Design review of the part built by this model. Coordinates are the model's own, in mm. A direction names the side the tool comes from. Give positions to 0.01 mm unless a question says otherwise; leave off trailing zeros. Order: outer loops, then holes, each group sorted by start corner. A loop starts at its lowest first (then second) coordinate and runs counter-clockwise, first axis right, second up. Notation, with made-up numbers: (43, 62.25) -> (83, 62.25) arc R23 ccw to (83, 70.25) -> close; hole circle Ø9 at (2, -24). An arc over 180 degrees is marked (long way). Answer in a Markdown table with one row per item. Add a question column.
```python
from build123d import *

# Parameters (mm, degrees)
BOSS_EXTRUDE1_DEPTH  = 60
CUT_EXTRUDE1_DEPTH   = 40
SKETCH11_W           = 2.5
SKETCH11_H           = 2.5
BOSS_EXTRUDE2_DEPTH  = 2.5
SKETCH14_W           = 3
SKETCH14_H           = 60
BOSS_EXTRUDE5_DEPTH  = 47
SKETCH12_R           = 1.125
BOSS_EXTRUDE3_DEPTH  = 6
CUT_EXTRUDE2_DEPTH   = 10
SKETCH16_W           = 100
SKETCH16_H           = 55
BOSS_EXTRUDE6_DEPTH  = 5
BOSS_EXTRUDE8_START  = -2
BOSS_EXTRUDE8_DEPTH  = 16
SKETCH19_W           = 2.25
SKETCH19_H           = 17
BOSS_EXTRUDE9_DEPTH  = 2.5
SKETCH20_W           = 100
SKETCH20_H           = 55
SKETCH20_W_2         = 59
SKETCH20_H_2         = 13.250841504
BOSS_EXTRUDE10_DEPTH = 5


with BuildPart() as part:
    # Sketch1 → Boss-Extrude1 (new body)
    with BuildSketch(Plane(origin=(0, 0, 0), x_dir=(1, 0, 0), z_dir=(0, 1, 0))):
        Polygon((40.01980198, -3.267326733), (40.01980198, 51.732673267), (35.01980198, 51.732673267), (35.01980198, 4.732673267), (-26.98019802, 4.732673267), (-26.98019802, 51.732673267), (-59.98019802, 51.732673267), (-59.98019802, -3.267326733), align=None)
    extrude(amount=BOSS_EXTRUDE1_DEPTH)

    # Sketch3 → Cut-Extrude1 (cut)
    with BuildSketch(Plane.ZY.offset(59.98019802)):
        with BuildLine():
            Line((-28.858094019, 44.125420752), (-51.732673267, 44.125420752))
            Line((-51.732673267, 44.125420752), (-51.732673267, 15.874579248))
            Line((-51.732673267, 15.874579248), (-28.858094019, 15.874579248))
            ThreePointArc((-28.858094019, 15.874579248), (-14.732673267, 30), (-28.858094019, 44.125420752))
        make_face()
    extrude(amount=-CUT_EXTRUDE1_DEPTH, mode=Mode.SUBTRACT)

    # Sketch11 → Boss-Extrude2 (add)
    with BuildSketch(Plane(origin=(0, 0, -14.732673267), x_dir=(-1, 0, 0), z_dir=(0, 0, -1))):
        with Locations((32.98019802, 30)):
            Rectangle(SKETCH11_W, SKETCH11_H)
    extrude(amount=BOSS_EXTRUDE2_DEPTH)

    # Sketch14 → Boss-Extrude5 (add)
    with BuildSketch(Plane(origin=(0, 0, -4.732673267), x_dir=(-1, 0, 0), z_dir=(0, 0, -1))):
        with Locations((25.48019802, 30)):
            Rectangle(SKETCH14_W, SKETCH14_H)
    extrude(amount=BOSS_EXTRUDE5_DEPTH)

    # Sketch12 → Boss-Extrude3 (add)
    with BuildSketch(Plane.ZY.offset(-35.01980198)):
        with Locations(Location((-36.858094019, 35.3, 0), (0, 0, 180))):
            Circle(SKETCH12_R)
        with Locations(Location((-36.858094019, 21.3, 0), (0, 0, 180))):
            Circle(SKETCH12_R)
    extrude(amount=BOSS_EXTRUDE3_DEPTH)

    # Sketch15 → Cut-Extrude2 (cut)
    with BuildSketch(Plane.ZY.offset(26.98019802)):
        with BuildLine():
            Line((-28.858094019, 35), (-51.732673267, 35))
            Line((-51.732673267, 35), (-51.732673267, 25))
            Line((-51.732673267, 25), (-28.858094019, 25))
            ThreePointArc((-28.858094019, 25), (-23.858094019, 30), (-28.858094019, 35))
        make_face()
    extrude(amount=-CUT_EXTRUDE2_DEPTH, mode=Mode.SUBTRACT)

    # Sketch16 → Boss-Extrude6 (add)
    with BuildSketch(Plane.XZ):
        with Locations((-9.98019802, -24.232673267)):
            Rectangle(SKETCH16_W, SKETCH16_H)
    extrude(amount=BOSS_EXTRUDE6_DEPTH)

    # Sketch18 → Boss-Extrude8 (add)
    with BuildSketch(Plane(origin=(0, 34.175, 0), x_dir=(-1, 0, 0), z_dir=(0, -1, 0)).offset(BOSS_EXTRUDE8_START)):
        Polygon((-35.01980198, 21.858094019), (-35.01980198, 9.965789174), (-29.01980198, 20.358094019), (-32.51980198, 20.358094019), (-32.51980198, 21.858094019), align=None)
    extrude(amount=BOSS_EXTRUDE8_DEPTH)

    # Sketch19 → Boss-Extrude9 (add)
    with BuildSketch(Plane.ZY.offset(-35.01980198)):
        with Locations((-36.858094019, 28.3)):
            Rectangle(SKETCH19_W, SKETCH19_H)
    extrude(amount=BOSS_EXTRUDE9_DEPTH)

    # Sketch20 → Boss-Extrude10 (add)
    with BuildSketch(Plane(origin=(0, 60, 0), x_dir=(1, 0, 0), z_dir=(0, 1, 0))):
        with Locations((-9.98019802, 24.232673267)):
            Rectangle(SKETCH20_W, SKETCH20_H)
        with Locations((5.51980198, 11.358094019)):
            Rectangle(SKETCH20_W_2, SKETCH20_H_2, mode=Mode.SUBTRACT)
    extrude(amount=BOSS_EXTRUDE10_DEPTH)


solid = part.part
```
1) Add section B-B, the plane y = 30. Write out the cut boundary in (x, z), and give its area (3 significant figures).
2) Mouldability with a two-part tool opening along X and no side actions: class faces 1 (the face through (34, 28, -35.733)), 2 (the face through (-11, -5, -24)), 3 (the face through (-23.98, 32, -23)), 4 (the face through (-34.23, 30, -16)) as +X half, -X half, draft (parallel to the pull), parting line (faces both ways), or undercut.
3) Add section C-C, the plane z = -31.5. Write out the cut boundary in (x, y).
4) Clearance check with flat-ended pins moving along their axes: P1, Ø8.5, axis at y = 32.5, z = -26.5, coming from the -X side; P2, Ø4, axis at x = 30, y = 31, coming from the -Z side; P3, Ø2.5, axis at y = 28.5, z = -36.5, coming from the -X side. State where each tip first meets the part, or that it passes through.
5) Add section A-A, the plane x = 1. Write out the cut boundary in (y, z), and give its area (3 significant figures).
6) Machinability: for faces 5 (the face through (-33, 31.25, -16)), 6 (the face through (32.06, 28.29, -15.09)), 7 (the face through (5, 62, -17.984)), which of the approach directions +Z, -Z, +X, -X, +Y, -Y give a long, thin tool a straight path to every point of the face, cutting with its end or side? Answer none if there is none.
7) For L1, parallel to X at y = 9.5, z = -25; L2, parallel to Y at x = -1, z = -35; L3, parallel to Y at x = -51, z = -39.5, list the stretches that pass through material, from the lowest coordinate up.
8) Add section D-D, the plane y = 56. Write out the cut boundary in (x, z), and give its area (3 significant figures).
Verdict:
| question | item | result |
|---|---|---|
| 1 | outline | (-59.98, -14.73) -> (-34.23, -14.73) -> (-34.23, -17.23) -> (-31.73, -17.23) -> (-31.73, -14.73) -> (-26.98, -14.73) -> (-26.98, -23.86) -> (-23.98, -23.86) -> (-23.98, -4.73) -> (35.02, -4.73) -> (35.02, -9.97) -> (29.02, -20.36) -> (32.52, -20.36) -> (32.52, -21.86) -> (35.02, -21.86) -> (35.02, -35.73) -> (32.52, -35.73) -> (32.52, -37.98) -> (35.02, -37.98) -> (35.02, -51.73) -> (40.02, -51.73) -> (40.02, 3.27) -> (-59.98, 3.27) -> close |
| 1 | area | 1,470 mm2 |
| 2 | face 1 | undercut |
| 2 | face 2 | draft |
| 2 | face 3 | undercut |
| 2 | face 4 | -X half |
| 3 | outline | (-59.98, -5) -> (40.02, -5) -> (40.02, 65) -> (-59.98, 65) -> (-59.98, 44.13) -> (-26.98, 44.13) -> (-26.98, 35) -> (-23.98, 35) -> (-23.98, 60) -> (35.02, 60) -> (35.02, 0) -> (-23.98, 0) -> (-23.98, 25) -> (-26.98, 25) -> (-26.98, 15.87) -> (-59.98, 15.87) -> close |
| 4 | P1 | stops at x = -26.98 |
| 4 | P2 | stops at z = -20.36 |
| 4 | P3 | stops at x = 32.52 |
| 5 | outline | (-5, -51.73) -> (0, -51.73) -> (0, -4.73) -> (65, -4.73) -> (65, 3.27) -> (-5, 3.27) -> close; (60, -51.73) -> (65, -51.73) -> (65, -17.98) -> (60, -17.98) -> close |
| 5 | area | 964 mm2 |
| 6 | face 5 | -Z, -X |
| 6 | face 6 | none |
| 6 | face 7 | +Y |
| 7 | L1 | x = -59.98 to -23.98, 35.02 to 40.02 |
| 7 | L2 | y = -5 to 0, 60 to 65 |
| 7 | L3 | y = -5 to 15.87, 44.13 to 65 |
| 8 | outline | (-59.98, -51.73) -> (-23.98, -51.73) -> (-23.98, -4.73) -> (35.02, -4.73) -> (35.02, -51.73) -> (40.02, -51.73) -> (40.02, 3.27) -> (-59.98, 3.27) -> close |
| 8 | area | 2,730 mm2 |
